Source: CAD feature listing. Evaluate the final solid. Frame: model axes, mm. A direction names the side the tool comes from. Round coordinates to 2 decimals unless told otherwise and drop trailing zeros. Order: outer loops, then holes, each group sorted by start corner. A loop starts at its lowest first (then second) coordinate and runs counter-clockwise, first axis right, second up. Notation, with made-up numbers: (25.5, 83.25) -> (56.5, 83.25) arc R19 cw to (56.5, 110.25) -> close; hole circle Ø7 at (45, -17.75). An arc over 180 degrees is marked (long way). Answer as CSV lines item,"result". Start each with the question number.
(1) Section query D-D (y = 108.5). Output: boundary loops of the cut face in (x, z).
(2) Section query A-A (y = 0). Output: boundary loops of the cut face in (x, z).
(3) Line query: line 1 along Z through (x, y) = (-102, 165); line 2 along Y through (x, z) = (-427.5, 414.5); line 3 along X through (y, z) = (241.5, 571). Output: solid intervals per line, ascending. Write a range as from..to.
(4) Contact query for flat-ended pins moving along their axis: P1, Ø2.5, axis at y = 272, z = 308.5, coming from the +X side; P2, Ø3, axis at x = -227, z = 561.5, coming from the -Y side; P3, Ø2.5, axis at y = 272, z = 623, coming from the -X side. Output: stop coordinate, or through.
(5) Section query B-B (y = 54). Output: boundary loops of the cut face in (x, z).
(6) Set-up query: faces 1 (the cylindrical face through (-12.973, -21.371, 493)), 2 (the flat face through (-113, 161, 980)). Return all of +Z, -Z, +X, -X, +Y, -Y with unobstructed straight access to the full face (end or side cutting, diameter ignored); none if empty.
(7) Section query C-C (z = 295). Count the separate pieces of the cut face and the enclosed holes in it, plus the area to 3 significant figures.
(8) Pull-direction query (Y, two-part tool) for faces 3 (the flat face through (-123, 192, 1000)), 4 (the flat face through (-406, 270, 493)), 5 (the cylindrical face through (-446.36, 233.14, 493)), 6 (the cylindrical face through (58.36, 134.64, 493.28)); classes: +Y half, -Y half, draft (parallel to the pull), parting line (faces both ways), or undercut.
```python
from build123d import *

# Parameters (mm, degrees)
SKETCH1_R           = 15
BOSS_EXTRUDE1_DEPTH = 1000
SKETCH2_W           = 13.606398545
SKETCH2_H           = 3.01775833
BOSS_EXTRUDE2_DEPTH = 1000
SHELL1_START        = 20
SHELL1_DEPTH        = 960


# Read off the part's stored shape, not the designer's step: Shell1
with BuildPart() as part:
    # Sketch1 → Boss-Extrude1 (new body)
    with BuildSketch(Plane.XY):
        with BuildLine():
            Line((90.647552146, 270), (-424.352447854, 270))
            ThreePointArc((-424.352447854, 270), (-446.003082949, 232.5), (-402.70181276, 232.5))
            Line((-402.70181276, 232.5), (-21.650635095, 12.5))
            ThreePointArc((-21.650635095, 12.5), (-12.5, -21.650635095), (21.650635095, -12.5))
            ThreePointArc((21.650635095, -12.5), (76.346217655, 123.817117551), (90.647552146, 270))
        make_face()
        with Locations((-424.352447854, 245)):
            Circle(SKETCH1_R, mode=Mode.SUBTRACT)
        Circle(SKETCH1_R, mode=Mode.SUBTRACT)
    extrude(amount=BOSS_EXTRUDE1_DEPTH)

    # Sketch2 → Boss-Extrude2 (add)
    with BuildSketch(Plane.XY.offset(1000)):
        with Locations((-381.021044878, 271.508879165)):
            Rectangle(SKETCH2_W, SKETCH2_H)
        with Locations((-351.021044878, 271.508879165)):
            Rectangle(SKETCH2_W, SKETCH2_H)
        with Locations((-321.021044878, 271.508879165)):
            Rectangle(SKETCH2_W, SKETCH2_H)
        with Locations((-291.021044878, 271.508879165)):
            Rectangle(SKETCH2_W, SKETCH2_H)
        with Locations((-261.021044878, 271.508879165)):
            Rectangle(SKETCH2_W, SKETCH2_H)
        with Locations((-231.021044879, 271.508879165)):
            Rectangle(SKETCH2_W, SKETCH2_H)
        with Locations((-201.021044879, 271.508879165)):
            Rectangle(SKETCH2_W, SKETCH2_H)
        with Locations((-171.021044878, 271.508879165)):
            Rectangle(SKETCH2_W, SKETCH2_H)
        with Locations((-141.021044878, 271.508879165)):
            Rectangle(SKETCH2_W, SKETCH2_H)
        with Locations((-111.021044879, 271.508879165)):
            Rectangle(SKETCH2_W, SKETCH2_H)
        with Locations((-81.021044879, 271.508879165)):
            Rectangle(SKETCH2_W, SKETCH2_H)
        with Locations((-51.021044879, 271.508879165)):
            Rectangle(SKETCH2_W, SKETCH2_H)
        with Locations((-21.021044878, 271.508879165)):
            Rectangle(SKETCH2_W, SKETCH2_H)
        with Locations((8.978955122, 271.508879165)):
            Rectangle(SKETCH2_W, SKETCH2_H)
        with Locations((38.978955122, 271.508879165)):
            Rectangle(SKETCH2_W, SKETCH2_H)
        with Locations((68.978955122, 271.508879165)):
            Rectangle(SKETCH2_W, SKETCH2_H)
    extrude(amount=-BOSS_EXTRUDE2_DEPTH)

    # Shell1 outline → Shell1 (cut)
    with BuildSketch(Plane.XY.offset(SHELL1_START)):
        with BuildLine():
            ThreePointArc((20.675289686, 28.240616077), (58.720352341, 136.205240665), (71.151752213, 250))
            Line((71.151752213, 250), (-389.711431703, 250))
            ThreePointArc((-389.711431703, 250), (-389.983130142, 238.385621722), (-394.041558722, 227.5))
            Line((-394.041558722, 227.5), (-30.310889132, 17.5))
            ThreePointArc((-30.310889132, 17.5), (-7.214665799, 34.248337148), (20.675289686, 28.240616077))
        make_face()
    extrude(amount=SHELL1_DEPTH, mode=Mode.SUBTRACT)


solid = part.part
```
Answer block:
1,outline,"(-187.93, 0) -> (72.36, 0) -> (72.36, 1000) -> (-187.93, 1000) -> (-187.93, 980) -> (51.57, 980) -> (51.57, 20) -> (-187.93, 20) -> close"
2,outline,"(-25, 0) -> (-15, 0) -> (-15, 1000) -> (-25, 1000) -> close; (15, 0) -> (28.64, 0) -> (28.64, 1000) -> (15, 1000) -> close"
3,line 1,"0..20, 980..1000"
3,line 2,"220.2..230.33, 259.67..269.8"
3,line 3,"-449.11..-438.94, -409.77..-389.53, 71.13..91.13"
4,P1,"x = 75.78"
4,P2,"y = 250"
4,P3,"x = -387.82"
5,outline,"(-93.53, 0) -> (53.96, 0) -> (53.96, 1000) -> (-93.53, 1000) -> (-93.53, 980) -> (32.35, 980) -> (32.35, 20) -> (-93.53, 20) -> close"
6,face 1,"+Z, -Z"
6,face 2,"none"
7,separate pieces,"1"
7,enclosed holes,"2"
7,area,"18,800 mm2"
8,face 3,"draft"
8,face 4,"+Y half"
8,face 5,"parting line"
8,face 6,"undercut"
